```python
from build123d import *

# Parameters (mm, degrees)
BOSS_EXTRUDE1_DEPTH      = 3
BOSS_EXTRUDE1_DEPTH_BACK = 3
CUT_EXTRUDE1_DEPTH       = 3
CUT_EXTRUDE1_DEPTH_BACK  = 3
SKETCH2_R                = 1.5
CUT_EXTRUDE3_DEPTH       = 3
CUT_EXTRUDE3_DEPTH_BACK  = 3
SKETCH4_R                = 1.5
FILLET1_R                = 5


with BuildPart() as part:
    # Sketch3 → Boss-Extrude1 (new, two sides: drawn at the far end of the back side and taken through both)
    with BuildSketch(Plane(origin=(0, 0, 0), x_dir=(1, 0, 0), z_dir=(0, 1, 0)).offset(-BOSS_EXTRUDE1_DEPTH_BACK)):
        Polygon((-3, 1.5), (-8, -2), (-14, -2), (-14, -5), (-8, -5), (-3, -1.5), (3, -1.5), (3, 1.5), align=None)
    extrude(amount=BOSS_EXTRUDE1_DEPTH + BOSS_EXTRUDE1_DEPTH_BACK)

    # Sketch2 → Cut-Extrude1 (cut, two sides: drawn at the far end of the back side and taken through both)
    with BuildSketch(Plane.XY.offset(-CUT_EXTRUDE1_DEPTH_BACK)):
        with BuildLine():
            ThreePointArc((0, 3), (2.121320344, 2.121320344), (3, 0))
            Line((3, 0), (3, 3))
            Line((3, 3), (0, 3))
        make_face()
        with BuildLine():
            ThreePointArc((3, 0), (2.121320338, -2.121320349), (-1.5e-08, -3))
            Line((-1.5e-08, -3), (3, -3))
            Line((3, -3), (3, 0))
        make_face()
        Circle(SKETCH2_R)
    extrude(amount=CUT_EXTRUDE1_DEPTH + CUT_EXTRUDE1_DEPTH_BACK, mode=Mode.SUBTRACT)

    # Sketch4 → Cut-Extrude3 (cut, two sides: drawn at the far end of the back side and taken through both)
    with BuildSketch(Plane.XY.offset(5).offset(-CUT_EXTRUDE3_DEPTH_BACK)):
        with BuildLine():
            ThreePointArc((-11, -3), (-13.121320344, -2.121320344), (-14, 0))
            Line((-14, 0), (-14, -3))
            Line((-14, -3), (-11, -3))
        make_face()
        with BuildLine():
            ThreePointArc((-14, 0), (-13.121320344, 2.121320344), (-11, 3))
            Line((-11, 3), (-14, 3))
            Line((-14, 3), (-14, 0))
        make_face()
        with Locations((-11, 0)):
            Circle(SKETCH4_R)
    extrude(amount=CUT_EXTRUDE3_DEPTH + CUT_EXTRUDE3_DEPTH_BACK, mode=Mode.SUBTRACT)

    # Fillet1
    fillet1_edges = [part.edges().sort_by_distance(p)[0] for p in [
        (-8, 0, 5),
        (-8, 0, 2),
        (-3, 0, -1.5),
        (-3, 0, 1.5),
    ]]
    fillet(fillet1_edges, radius=FILLET1_R)


solid = part.part
```
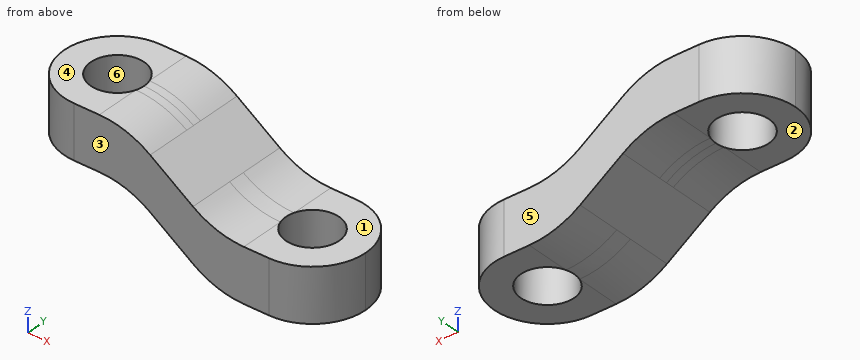
Build history of the part. All positions in model axes, mm. Face numbers are marked on the shaded views. A direction names the side the tool comes from. Round coordinates to 2 decimals unless told otherwise and drop trailing zeros. Write each loop counter-clockwise with the first axis right and the second up, starting at its lowest first coordinate (ties: lowest second). Pieces come first, ordered by that corner, then holes.
1) Drill centre lines: probe 1 along Y at (x, z) = (-11, 2.95); probe 2 along Z at (x, y) = (-9.5, 2.25); probe 3 along Z at (x, y) = (1.5, 2). Where is each one in solid material? Low to high.
2) Band-saw the part on B-B, the plane z = 3.25. List the corners of the cut face in (x, y), and give its area (3 significant figures).
3) Mould opens along Y. For the marked faces 4, 5 and 6 say: +Y half, -Y half, draft (parallel to the pull), parting line (faces both ways), or undercut.
4) 3-axis set-ups, long thin cutter, end or side, ignore diameter. For the marked faces 1, 2 and 3: which of +Z, -Z, +X, -X, +Y, -Y reach the whole face in a straight line?
5) Band-saw the part on D-D, the plane y = 2.5. List the corners of the cut face in (x, z), and give its area (4 significant figures).
6) Band-saw the part on A-A, the plane x = -0.75. List the corners of the cut face in (y, z).
7) Pin check, flat tips, straight feed: pin 1 (2 mm diameter, centred on x = -12.5, y = 1.5, fed in from -Z); pin 2 (2 mm diameter, centred on y = 1.5, z = -0.5, fed in from -X); pin 3 (1 mm diameter, centred on y = 1, z = 3, fed in from +X). Stop position of each tip, or through.
8) Band-saw the part on C-C, the plane x = -9.75. List the corners of the cut face in (y, z), and give its area (3 significant figures).
Ans:
1. probe 1: y = -3 to -1.5, 1.5 to 3
1. probe 2: z = 2 to 5
1. probe 3: z = -1.5 to 1.5
2. outline: (-11, -3) - (-5.5, -3) - (-5.5, 3) - (-11, 3) arc R3 ccw to start; hole circle Ø3 at (-11, 0)
2. area: 40.1 mm2
3. face 4: draft
3. face 5: +Y half
3. face 6: undercut
4. face 1: +Z, +X, +Y, -Y
4. face 2: -Z, -X, +Y, -Y
4. face 3: +Z, -Z, +X, -X, -Y
5. outline: (-12.66, 2) - (-9.58, 2) arc R5 cw to (-6.71, 1.1) - (-4.29, -0.6) arc R5 ccw to (-1.42, -1.5) - (1.66, -1.5) - (1.66, 1.5) - (-1.42, 1.5) arc R5 cw to (-4.29, 2.4) - (-6.71, 4.1) arc R5 ccw to (-9.58, 5) - (-12.66, 5) - close
5. area: 42.95 mm2
6. outline: (-3, -1.5) - (-1.3, -1.5) - (-1.3, 1.5) - (-3, 1.5) - close; (1.3, -1.5) - (3, -1.5) - (3, 1.5) - (1.3, 1.5) - close
7. pin 1: stops at z = 2
7. pin 2: stops at x = -5.86
7. pin 3: stops at x = -4.43
8. outline: (-3, 2) - (-0.83, 2) - (-0.83, 5) - (-3, 5) - close; (0.83, 2) - (3, 2) - (3, 5) - (0.83, 5) - close
8. area: 13.0 mm2
